Autodesk Inventor part; units mm, degrees
ref_plane "YZ Plane" through (0, 0, 0) normal (1, 0, 0) x (0, 1, 0)
ref_plane "XZ Plane" through (0, 0, 0) normal (0, 1, 0) x (-1, 0, 0)
ref_plane "XY Plane" through (0, 0, 0) normal (0, 0, 1) x (1, 0, 0)
sketch "Sketch1" plane through (0, 0, 0) normal (0, 1, 0) x (-1, 0, 0)
  line L0 (-14.3815, 30) -> (14.3815, 30)
  line L1 (14.3815, 30) -> (14.3815, -30)
  line L2 (14.3815, -30) -> (-14.3815, -30)
  line L3 (-14.3815, -30) -> (-14.3815, 30)
  line L4 (-14.3815, 30) -> (14.3815, -30) construction
  line L5 (14.3815, 30) -> (-14.3815, -30) construction
  point P0 (0, 0)
  dimension "d2" = 60
  dimension "d3" = 28.763
extrude "Extrusion1" add sketch "Sketch1" along normal mid plane 2
sketch "Sketch2" plane through (0, 1, 0) normal (0, 1, 0) x (1, 0, 0)
  circle A0 centre (0, 0) radius 5
  dimension "d4" = 10
extrude "Extrusion2" cut sketch "Sketch2" against normal through all
sketch "Sketch3" plane through (0, 1, 0) normal (0, 1, 0) x (1, 0, 0)
  line L0 (0, 0) -> (0, 30) construction
  line L1 (-14.3815, 30) -> (14.3815, 30) construction
  line L2 (0, 0) -> (0, -30) construction
  line L3 (14.3815, -30) -> (-14.3815, -30) construction
  point P0 (0, -15)
  point P1 (0, 15)
hole "Hole1" at (0, 1, 15) at (0, 1, -15) direction (0, -1, 0) diameter 4.305 end through all
sketch "Sketch4" plane through (0, -1, 0) normal (0, -1, 0) x (1, 0, 0)
  circle A0 centre (-12.3815, 28) radius 0.975
  circle A1 centre (-12.3815, -28) radius 0.975
  circle A2 centre (12.3815, -28) radius 0.975
  circle A3 centre (12.3815, 28) radius 0.975
  line L0 (-14.3815, 30) -> (-14.3815, -30)
  line L1 (14.3815, 30) -> (-14.3815, 30)
  line L2 (14.3815, -30) -> (14.3815, 30)
  line L3 (-14.3815, -30) -> (14.3815, -30)
  point P0 (0, 0)
  dimension "d14" = 1.95
  dimension "d15" = 2
  dimension "d16" = 2
  dimension "d17" = 2
  dimension "d18" = 2
extrude "Extrusion3" add sketch "Sketch4" along normal blind 2 contours A0 | A1 | A2 | A3
fillet "Fillet1" radius 2 4 edges at (14.3815, 0, 30) (-14.3815, 0, 30) (-14.3815, 0, -30) (14.3815, 0, -30)
equation "\"d16\" = d15"
equation "\"d17\" = d15"
equation "\"d18\" = d15"
properties part number "GearCoverTop"
The model under review builds one solid part; all positions refer to its coordinate system, in mm. A direction names the side the tool comes from. Give positions to 0.01 mm unless a question says otherwise; leave off trailing zeros. Order: outer loops, then holes, each group sorted by start corner. A loop starts at its lowest first (then second) coordinate and runs counter-clockwise, first axis right, second up. Notation, with made-up numbers: M -28.5,62 L 22.5,62 A22 ccw 22.5,88 Z; hole C 34,-2 d11. An arc over 180 degrees is marked long. Answer in a Markdown table with one row per item. Add a question column.
1. Mouldability with a two-part tool opening along Z and no side actions: class faces 1 (the cylindrical face through (12.255, -1.986, 27.033)), 2 (the cylindrical face through (-0.65, -0.01, -12.95)), 3 (the cylindrical face through (13.81, 0.01, -29.4)), 4 (the flat face through (12, -3, 28)) as released by +Z, released by -Z, zero draft, split by the parting line, or undercut.
2. Add section B-B on x = 0. State the section outline as (y, z) points.
3. To check wall thickness, follow line 1 along Z through (x, y) = (0, 0.6); line 2 along X through (y, z) = (-0.6, 0); line 3 along X through (y, z) = (0.3, -15). State the ranges of each line that lie inside material, in increasing order.
4. For pin 1 Ø11.5 at (x, z) = (0, 0) entering from -Y; pin 2 Ø4 at (x, z) = (0, -15) entering from +Y, all flat-tipped, find the tip position at first contact; note any pin that passes through.
5. Add section C-C on y = -1.6. Count the separate pieces of the cut face and the enclosed holes in it, plus the area to 3 significant figures.
6. Add section D-D on z = 15. State the section outline as (x, y) points.
7. Machinability: for faces 5 (the cylindrical face through (-0.09, -0.01, 12.85)), 6 (the cylindrical face through (-12.508, -1.986, 27.033)), which of the approach directions +Z, -Z, +X, -X, +Y, -Y give a long, thin tool a straight path to every point of the face, cutting with its end or side? Answer none if there is none.
8. Add section A-A on z = 0. State the section outline as (x, y) points, plus the area to 3 significant figures.
The answers:
| question | item | result |
|---|---|---|
| 1 | face 1 | undercut |
| 1 | face 2 | undercut |
| 1 | face 3 | released by -Z |
| 1 | face 4 | zero draft |
| 2 | outline | M -1,-30 L 1,-30 L 1,-17.15 L -1,-17.15 Z; M -1,-12.85 L 1,-12.85 L 1,-5 L -1,-5 Z; M -1,5 L 1,5 L 1,12.85 L -1,12.85 Z; M -1,17.15 L 1,17.15 L 1,30 L -1,30 Z |
| 3 | line 1 | -30 to -17.15, -12.85 to -5, 5 to 12.85, 17.15 to 30 |
| 3 | line 2 | -14.38 to -5, 5 to 14.38 |
| 3 | line 3 | -14.38 to -2.15, 2.15 to 14.38 |
| 4 | pin 1 | y = -1 |
| 4 | pin 2 | through |
| 5 | separate pieces | 4 |
| 5 | enclosed holes | 0 |
| 5 | area | 11.9 mm2 |
| 6 | outline | M -14.38,-1 L -2.15,-1 L -2.15,1 L -14.38,1 Z; M 2.15,-1 L 14.38,-1 L 14.38,1 L 2.15,1 Z |
| 7 | face 5 | +Y, -Y |
| 7 | face 6 | -Y |
| 8 | outline | M -14.38,-1 L -5,-1 L -5,1 L -14.38,1 Z; M 5,-1 L 14.38,-1 L 14.38,1 L 5,1 Z |
| 8 | area | 37.5 mm2 |
